Here's how the part is built. I have some questions about the finished solid (model axes, mm). Face numbers are marked on the shaded views. A direction names the side the tool comes from. Round coordinates to 2 decimals unless told otherwise and drop trailing zeros. Write each loop counter-clockwise with the first axis right and the second up, starting at its lowest first coordinate (ties: lowest second). Pieces come first, ordered by that corner, then holes. Notation, with made-up numbers: (81, 5.25) -> (117, 5.25) arc R12 cw to (117, 18.25) -> close; hole circle Ø2 at (24.5, 37). An arc over 180 degrees is marked (long way). Put each result on its own line as item: value. Start each with the question number.
1. Suppose I cut it at B-B (x = 8). Please give me the cut outline in (y, z), then the cut area to 3 significant figures.
2. Which directions (+Z, -Z, +X, -X, +Y, -Y) give clear straight access to the entire face, cutting with the end or side of a thin tool? Please do the marked faces 1, 2, 3, 4 and 5.
3. Suppose I cut it at A-A (y = 19.5). Please give me the cut outline in (x, z).
4. For pin 1 (2 mm diameter, centred on x = 8.5, y = 3.5, fed in from -Z); pin 2 (3 mm diameter, centred on x = 2, y = 17.5, fed in from +Z); pin 3 (1 mm diameter, centred on x = 2, z = -7, fed in from +Y); pin 4 (2.5 mm diameter, centred on y = 19.1, z = 0, fed in from +X), each with a flat end and sliding along its axis, tell me the tip position at first contact or that it passes through.
5. We'd pull the mould along Z, two halves only. Please class the marked faces 6, 7 and 8: +Z half, -Z half, draft (parallel to the pull), parting line (faces both ways), or undercut.
6. Suppose I cut it at C-C (z = -7.25). Please give me the cut outline in (x, y), then the cut area to 3 significant figures.
7. Suppose I cut it at D-D (x = 5). Please give me the cut outline in (y, z).
8. I need wall thicknesses on probe 1 along Y at (x, z) = (3.75, 0); probe 2 along Y at (x, z) = (7.95, 0); probe 3 along Z at (x, y) = (8.85, 10). Which ranges of each line are inside material? Lowest first, please. Write a range as from..to.
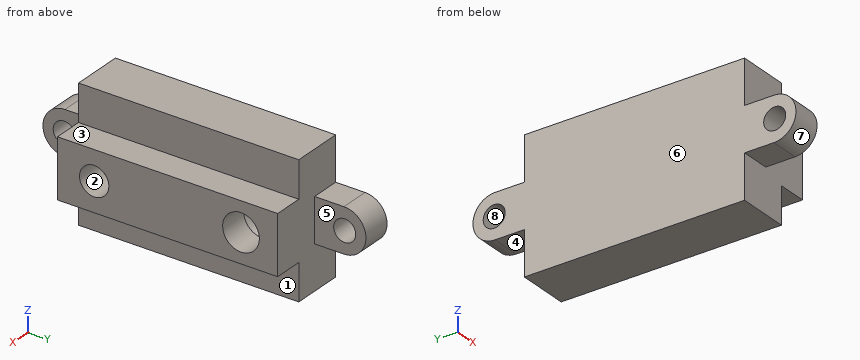
Autodesk Inventor part; units mm, degrees
ref_plane "YZ Plane" through (0, 0, 0) normal (1, 0, 0) x (0, 1, 0)
ref_plane "XZ Plane" through (0, 0, 0) normal (0, 1, 0) x (-1, 0, 0)
ref_plane "XY Plane" through (0, 0, 0) normal (0, 0, 1) x (1, 0, 0)
sketch "Skizze1" plane through (0, 0, 0) normal (1, 0, 0) x (0, 1, 0)
  line L0 (-15, -9) -> (15, -9)
  line L1 (15, -9) -> (15, 9)
  line L2 (15, 9) -> (-15, 9)
  line L3 (-15, 9) -> (-15, -9)
  line L4 (-15, -9) -> (15, 9) construction
  line L5 (15, -9) -> (-15, 9) construction
  point P0 (0, 0)
  dimension "d0" = 30
  dimension "d1" = 18
extrude "Extrusion1" add sketch "Skizze1" along normal blind 7
sketch "Skizze2" plane through (7, 0, 0) normal (1, 0, 0) x (0, 0, -1)
  line L0 (4, -15) -> (-4, -15)
  line L1 (-4, -15) -> (-4, 15)
  line L2 (-4, 15) -> (4, 15)
  line L3 (4, 15) -> (4, -15)
  line L4 (4, -15) -> (-4, 15) construction
  line L5 (-4, -15) -> (4, 15) construction
  point P0 (0, 0)
  dimension "d4" = 8
  dimension "d5" = 30
extrude "Extrusion2" add sketch "Skizze2" along normal blind 4
sketch "Skizze3" plane through (11, 0, 0) normal (1, 0, 0) x (0, 0, -1)
  point P0 (0, 0)
  point P1 (0.0058, 10)
  dimension "d24" = 10
hole "Bohrung1" at (11, 10, -0.0058) direction (-1, 0, 0) diameter 5 depth 4 tip angle 118
sketch "Skizze4" plane through (11, 0, 0) normal (1, 0, 0) x (0, 0, -1)
  line L0 (-4, -15) -> (4, -15)
  point P0 (0, 0)
  point P1 (0, -10)
  dimension "d22" = 0
  dimension "d23" = 5
hole "Bohrung2" at (11, -10, 0) direction (-1, 0, 0) diameter 4 depth 4 tip angle 118
sketch "Skizze5" plane through (0, 0, 0) normal (-1, 0, 0) x (0, 0, 1)
  line L0 (-9, 15) -> (9, 15)
  line L1 (-3, 15) -> (-3, 19)
  line L2 (-3, 15) -> (1, 15) construction
  line L3 (3, 15) -> (3, 19)
  line L4 (-3, 15) -> (3, 15)
  arc A0 (3, 19) -> (-3, 19) centre (0, 19) ccw
  point P0 (0, 0)
  point P1 (-3, 17)
  dimension "d25" = 4
  dimension "d26" = 90
  dimension "d27" = 3
  dimension "d28" = 3
extrude "Extrusion3" add sketch "Skizze5" against normal blind 4
sketch "Skizze6" plane through (4, 0, 0) normal (1, 0, 0) x (0, 0, -1)
  point P0 (0, 0)
  point P1 (0, 19.1025)
  dimension "d38" = 0
hole "Bohrung3" at (4, 19.1025, 0) direction (-1, 0, 0) diameter 3 depth 4 tip angle 118
mirror "Spiegeln1" about plane through (0, 0, 0) normal (0, 1, 0) of "Extrusion3", "Bohrung3"
properties part number "InfraSensor"
Verdict:
1. outline: (-15, -4) -> (15, -4) -> (15, 4) -> (-15, 4) -> close; hole circle Ø4 at (-10, 0); hole circle Ø5 at (10, -0.01)
1. area: 208 mm^2
2. face 1: -Z, +X, +Y, -Y
2. face 2: +X
2. face 3: +Z, +X, +Y, -Y
2. face 4: -Z, +X, -X, +Y
2. face 5: +Z, -Z, +X, +Y
3. outline: (0, -2.96) -> (4, -2.96) -> (4, -1.45) -> (0, -1.45) -> close; (0, 1.45) -> (4, 1.45) -> (4, 2.96) -> (0, 2.96) -> close
4. pin 1: stops at z = -4
4. pin 2: stops at z = 3
4. pin 3: stops at y = 15
4. pin 4: passes through
5. face 6: draft
5. face 7: parting line
5. face 8: undercut
6. outline: (0, -15) -> (7, -15) -> (7, 15) -> (0, 15) -> close
6. area: 210 mm^2
7. outline: (-15, -9) -> (15, -9) -> (15, 9) -> (-15, 9) -> close
8. probe 1: y = -22..-20.6, -17.6..17.6, 20.6..22
8. probe 2: y = -15..-12, -8..7.5, 12.5..15
8. probe 3: z = -4..-2.51, 2.49..4
